```python
from build123d import *

# Parameters (mm, degrees)
SKETCH_1_W          = 50
SKETCH_1_H          = 30
EXTRUDE_1_DEPTH     = 70
SKETCH_2_R          = 9.55
CUT_EXTRUDE_1_DEPTH = 120
CUT_EXTRUDE_START   = 15
SKETCH_3_W          = 15.6
SKETCH_3_H          = 15.6
CUT_EXTRUDE_3_DEPTH = 1
SKETCH_4_W          = 2.75
SKETCH_4_H          = 15.6
CUT_EXTRUDE_4_DEPTH = 3


with BuildPart() as part:
    # 草图1 → 凸台-拉伸1 (new body)
    with BuildSketch(Plane(origin=(0, 0, 0), x_dir=(1, 0, 0), z_dir=(0, 1, 0))):
        Rectangle(SKETCH_1_W, SKETCH_1_H)
    extrude(amount=EXTRUDE_1_DEPTH)

    # 草图2 → 切除-拉伸1 (cut)
    with BuildSketch(Plane.XZ):
        with Locations(Location((0, 0, 0), (0, 0, 270))):
            Circle(SKETCH_2_R)
    extrude(amount=-CUT_EXTRUDE_1_DEPTH, mode=Mode.SUBTRACT)

    # 草图3 → 切除-拉伸3 (cut)
    with BuildSketch(Plane.XY.offset(CUT_EXTRUDE_START)):
        with Locations((0, 52.2)):
            Rectangle(SKETCH_3_W, SKETCH_3_H)
    extrude(amount=-CUT_EXTRUDE_3_DEPTH, mode=Mode.SUBTRACT)

    # 草图4 → 切除-拉伸4 (cut)
    with BuildSketch(Plane.XY.offset(14)):
        with Locations((-6.425, 52.2)):
            Rectangle(SKETCH_4_W, SKETCH_4_H)
        with Locations((6.425, 52.2)):
            Rectangle(SKETCH_4_W, SKETCH_4_H)
    extrude(amount=-CUT_EXTRUDE_4_DEPTH, mode=Mode.SUBTRACT)


solid = part.part
```
Could you check a few things on this model? Use its own coordinates, in mm. A direction names the side the tool comes from. Give positions to 0.01 mm unless a question says otherwise; leave off trailing zeros. Write each loop counter-clockwise with the first axis right and the second up, starting at its lowest first coordinate (ties: lowest second). Pieces come first, ordered by that corner, then holes. Notation, with made-up numbers: (44, 73.5) -> (48, 73.5) arc R14 cw to (48, 91.5) -> close; hole circle Ø2 at (72, 71.5). An arc over 180 degrees is marked (long way). Write each question's results on one line, items separated by ' | '.
1. I want a section at D-D, the plane z = 13. Write out the boundary of the cut face in (x, y), then the cut area to 3 significant figures.
Check sheet entries:
outline: (-25, 0) -> (25, 0) -> (25, 70) -> (-25, 70) -> close; hole (-7.8, 44.4) -> (-5.05, 44.4) -> (-5.05, 60) -> (-7.8, 60) -> close; hole (5.05, 44.4) -> (7.8, 44.4) -> (7.8, 60) -> (5.05, 60) -> close | area: 3,410 mm²
2. I want a section at B-B, the plane x = 0. Write out the boundary of the cut face in (y, z), then the cut area to 3 significant figures.
Check sheet entries:
outline: (0, -15) -> (70, -15) -> (70, -9.55) -> (0, -9.55) -> close; (0, 9.55) -> (70, 9.55) -> (70, 15) -> (60, 15) -> (60, 14) -> (44.4, 14) -> (44.4, 15) -> (0, 15) -> close | area: 747 mm²
3. I need wall thicknesses on L1, parallel to Z at x = 5.5, y = 59; L2, parallel to X at y = 30, z = 0; L3, parallel to Z at x = 5.5, y = 4.5. Which ranges of each line are inside material? Lowest first, please.
Check sheet entries:
L1: z = -15 to -7.81, 7.81 to 11 | L2: x = -25 to -9.55, 9.55 to 25 | L3: z = -15 to -7.81, 7.81 to 15
4. I want a section at A-A, the plane z = 0. Write out the boundary of the cut face in (x, y), then the cut area to 3 significant figures.
Check sheet entries:
outline: (-25, 0) -> (-9.55, 0) -> (-9.55, 70) -> (-25, 70) -> close; (9.55, 0) -> (25, 0) -> (25, 70) -> (9.55, 70) -> close | area: 2,160 mm²
5. If we mould it in two halves opening along Y, with no side actions, what happens to faces 3 (the flat face through (0, 0, -10)), 4 (the flat face through (0, 70, -10)), 5 (the flat face through (0, 35, 15)), 6 (the flat face through (-5.05, 52, 13))? For each: released by +Y, released by -Y, zero draft, split by the parting line, or undercut.
Check sheet entries:
face 3: released by -Y | face 4: released by +Y | face 5: zero draft | face 6: undercut
6. I want a section at C-C, the plane y = 43.5. Write out the boundary of the cut face in (x, z), then the cut area to 3 significant figures.
Check sheet entries:
outline: (-25, -15) -> (25, -15) -> (25, 15) -> (-25, 15) -> close; hole circle Ø19.1 at (0, 0) | area: 1,210 mm²
7. On a 3-axis mill with a long thin cutter (end or side, diameter ignored), from which of +Z, -Z, +X, -X, +Y, -Y can I reach the whole of each face in a straight line? I mean faces 1 (the flat face through (-6, 52, 11)), 2 (the flat face through (0, 35, -15)). Say none if no direction works.
Check sheet entries:
face 1: +Z | face 2: -Z, +X, -X, +Y, -Y
8. Will these pins go through, and if not, where does the flat tip stop? pin 1 Ø8 at (x, y) = (-2, 55) entering from +Z; pin 2 Ø0.8 at (x, y) = (6, 54) entering from +Z.
Check sheet entries:
pin 1: stops at z = 14 | pin 2: stops at z = 11
